Geometry: final body of the model. Coordinates: model frame, mm. Face numbers are marked on the shaded views. A direction names the side the tool comes from. Give positions to 0.01 mm unless a question says otherwise; leave off trailing zeros. Write each loop counter-clockwise with the first axis right and the second up, starting at its lowest first coordinate (ties: lowest second). Pieces come first, ordered by that corner, then holes.
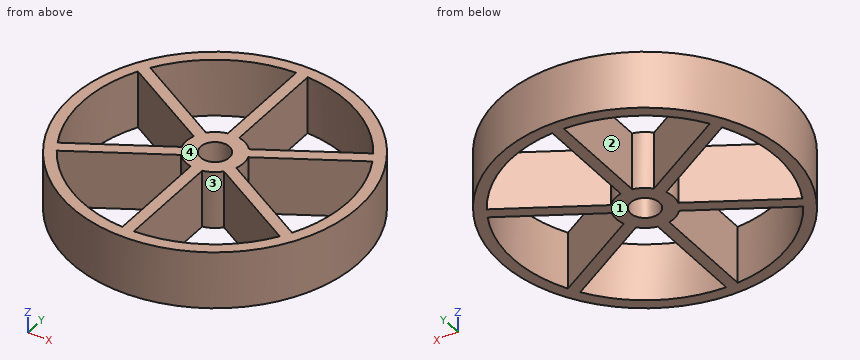
Autodesk Inventor part; units mm, degrees
ref_plane "YZ Plane" through (0, 0, 0) normal (1, 0, 0) x (0, 1, 0)
ref_plane "XZ Plane" through (0, 0, 0) normal (0, 1, 0) x (-1, 0, 0)
ref_plane "XY Plane" through (0, 0, 0) normal (0, 0, 1) x (1, 0, 0)
sketch "スケッチ1" plane through (0, 0, 0) normal (0, 0, 1) x (1, 0, 0)
  circle A0 centre (0, 0) radius 25
  circle A1 centre (0, 0) radius 23
  circle A2 centre (0, 0) radius 5
  circle A3 centre (0, 0) radius 2.5
  dimension "d0" = 50
  dimension "d1" = 2
  dimension "d2" = 10
  dimension "d3" = 5
extrude "押し出し1" add sketch "スケッチ1" along normal blind 10
sketch "スケッチ2" plane through (0, 0, 0) normal (0, 0, 1) x (1, 0, 0)
  line L0 (-1, 2.5) -> (1, 2.5)
  line L1 (1, 2.5) -> (1, 23)
  line L2 (1, 23) -> (-1, 23)
  line L3 (-1, 23) -> (-1, 2.5)
  circle A0 centre (0, 0) radius 23
  circle A1 centre (0, 0) radius 2.5
  point P0 (0, 2.5)
  point P1 (-1, 22.9783)
  point P2 (1, 22.9783)
  dimension "d6" = 2
extrude "押し出し2" add sketch "スケッチ2" along normal blind 10 contours L3 A0 L1 L0 picked at (-0.6667, 9.3261)
pattern_circular "円形状パターン1" count 6 over 360 about axis through (0, 0, -10) along (0, 0, 1) of "押し出し2"
properties part number "Wheel-D50"
Q1. Section C-C on z = 4.25. Output: boundary loops of the cut face in (x, y).
Filled sheet:
outline: circle Ø50 at (0, 0); hole (-20.4, -10.62) - (-4.74, -1.58) arc R5 cw to (-4.74, 1.58) - (-20.4, 10.62) arc R23 ccw to start; hole (-19.4, -12.36) arc R23 ccw to (-1, -22.98) - (-1, -4.9) arc R5 cw to (-3.74, -3.32) - close; hole (-19.4, 12.36) - (-3.74, 3.32) arc R5 cw to (-1, 4.9) - (-1, 22.98) arc R23 ccw to start; hole circle Ø5 at (0, 0); hole (1, -22.98) arc R23 ccw to (19.4, -12.36) - (3.74, -3.32) arc R5 cw to (1, -4.9) - close; hole (1, 4.9) arc R5 cw to (3.74, 3.32) - (19.4, 12.36) arc R23 ccw to (1, 22.98) - close; hole (4.74, -1.58) - (20.4, -10.62) arc R23 ccw to (20.4, 10.62) - (4.74, 1.58) arc R5 cw to start
Q2. Ray query, line 1 along Y through (x, z) = (-9, 4); line 2 along X through (y, z) = (2, 5.5); line 3 along Y through (x, z) = (0, 7.5). Return the intervals inside material, ascending.
Filled sheet:
line 1: y = -23.32 to -21.17, -6.35 to -4.04, 4.04 to 6.35, 21.17 to 23.32
line 2: x = -24.92 to -22.91, -5.46 to -1.5, 1.5 to 5.46, 22.91 to 24.92
line 3: y = -25 to -2.5, 2.5 to 25
Q3. Access query for the marked faces 3 and 4. Directions: +Z, -Z, +X, -X, +Y, -Y. A direction counts if a zero-diameter tool reaches every point of the face in a straight line with its end or side. Return the directions, or none.
Filled sheet:
face 3: +Z, -Z
face 4: +Z, +X, -X, +Y, -Y
Q4. Section B-B on y = 0. Output: boundary loops of the cut face in (x, z), plus the area to 3 significant figures.
Filled sheet:
outline: (-25, 0) - (-23, 0) - (-23, 10) - (-25, 10) - close; (-5, 0) - (-2.5, 0) - (-2.5, 10) - (-5, 10) - close; (2.5, 0) - (5, 0) - (5, 10) - (2.5, 10) - close; (23, 0) - (25, 0) - (25, 10) - (23, 10) - close
area: 90.0 mm2
Q5. Section A-A on x = 0. Output: boundary loops of the cut face in (y, z), plus the area to 3 significant figures.
Filled sheet:
outline: (-25, 0) - (-2.5, 0) - (-2.5, 10) - (-25, 10) - close; (2.5, 0) - (25, 0) - (25, 10) - (2.5, 10) - close
area: 450 mm2
Q6. Section D-D on x = -10.5. Output: boundary loops of the cut face in (y, z).
Filled sheet:
outline: (-22.69, 0) - (-20.46, 0) - (-20.46, 10) - (-22.69, 10) - close; (-7.22, 0) - (-4.91, 0) - (-4.91, 10) - (-7.22, 10) - close; (4.91, 0) - (7.22, 0) - (7.22, 10) - (4.91, 10) - close; (20.46, 0) - (22.69, 0) - (22.69, 10) - (20.46, 10) - close
Q7. Pin query (flat end, axial travel): P1, Ø3, axis at y = 3.5, z = 5.5, coming from the -X side; P2, Ø2, axis at y = -8.5, z = 4, coming from the +X side; P3, Ø6, axis at x = -4.5, z = 8.5, coming from the -Y side. Return the tip coordinate at first contact, or that it passes through.
Filled sheet:
P1: stops at x = -24.92
P2: stops at x = 23.85
P3: stops at y = -24.95
Q8. Pull-direction query (Y, two-part tool) for the marked faces 1 and 2; classes: released by +Y, released by -Y, zero draft, split by the parting line, or undercut.
Filled sheet:
face 1: zero draft
face 2: undercut
